Geometry check sheet. Reference: the model listing, model coordinates, mm. A direction names the side the tool comes from. Coordinates: 2 decimals unless noted, no trailing zeros. Write each loop counter-clockwise with the first axis right and the second up, starting at its lowest first coordinate (ties: lowest second). Pieces come first, ordered by that corner, then holes. Notation, with made-up numbers: M 30.25,76 L 40.25,76 A17 cw 40.25,100 Z; hole C 20,25 d7. An arc over 180 degrees is marked long. Write each question's results on one line, items separated by ' | '.
```python
from build123d import *

# Parameters (mm, degrees)
SKETCH_1_W                       = 400
SKETCH_1_H                       = 135
SKETCH_1_R                       = 3
SM_BASE_FLANGE_1_DEPTH           = 0.7
SM_EDGE_FLANGE_1_STRIP_W         = 3.2
SM_EDGE_FLANGE_1_STRIP_H         = 0.7
SM_EDGE_FLANGE_1_STRIP_CUT_DEPTH = 400
SM_EDGE_FLANGE_1_DEPTH           = 400
SM_EDGE_FLANGE_2_STRIP_W         = 3.2
SM_EDGE_FLANGE_2_STRIP_H         = 0.7
SM_EDGE_FLANGE_2_STRIP_CUT_DEPTH = 400
SM_EDGE_FLANGE_2_DEPTH           = 400


# Sheet-metal steps are written as plain solids
with BuildPart() as part:
    # Sketch 1 → 基体-法兰1 (new body)
    with BuildSketch(Plane(origin=(0, 0, 0), x_dir=(1, 0, 0), z_dir=(0, 1, 0))):
        Rectangle(SKETCH_1_W, SKETCH_1_H)
        with Locations(Location((-194.5, -60.5, 0), (0, 0, 270))):
            Circle(SKETCH_1_R, mode=Mode.SUBTRACT)
        with Locations(Location((-194.5, -10.5, 0), (0, 0, 270))):
            Circle(SKETCH_1_R, mode=Mode.SUBTRACT)
        with Locations(Location((-194.5, -0.5, 0), (0, 0, 270))):
            Circle(SKETCH_1_R, mode=Mode.SUBTRACT)
        with Locations(Location((-194.5, 49.5, 0), (0, 0, 270))):
            Circle(SKETCH_1_R, mode=Mode.SUBTRACT)
        with Locations(Location((0, -10.5, 0), (0, 0, 270))):
            Circle(SKETCH_1_R, mode=Mode.SUBTRACT)
        with Locations(Location((0, -0.5, 0), (0, 0, 270))):
            Circle(SKETCH_1_R, mode=Mode.SUBTRACT)
        with Locations(Location((194.5, -60.5, 0), (0, 0, 90))):
            Circle(SKETCH_1_R, mode=Mode.SUBTRACT)
        with Locations(Location((194.5, -10.5, 0), (0, 0, 90))):
            Circle(SKETCH_1_R, mode=Mode.SUBTRACT)
        with Locations(Location((194.5, -0.5, 0), (0, 0, 90))):
            Circle(SKETCH_1_R, mode=Mode.SUBTRACT)
        with Locations(Location((194.5, 49.5, 0), (0, 0, 90))):
            Circle(SKETCH_1_R, mode=Mode.SUBTRACT)
    extrude(amount=-SM_BASE_FLANGE_1_DEPTH)

    # 边线-法兰1 strip (across the edge) → 边线-法兰1 strip cut (cut)
    with BuildSketch(Plane(origin=(-200, -0.7, -67.5), x_dir=(0, 0, 1), z_dir=(1, 0, 0))):
        with Locations((-0.7, -0.35)):
            Rectangle(SM_EDGE_FLANGE_1_STRIP_W, SM_EDGE_FLANGE_1_STRIP_H)
    extrude(amount=SM_EDGE_FLANGE_1_STRIP_CUT_DEPTH, mode=Mode.SUBTRACT)

    # 边线-法兰1 section (across the edge) → 边线-法兰1 (add)
    with BuildSketch(Plane(origin=(-200, -0.7, -67.5), x_dir=(0, 0, 1), z_dir=(1, 0, 0))):
        with BuildLine():
            Line((0, 0.2), (0, 5.3))
            Line((0, 5.3), (0.7, 5.3))
            Line((0.7, 5.3), (0.7, 0.2))
            ThreePointArc((0.7, 0.2), (0.758578644, 0.058578644), (0.9, 0))
            Line((0.9, 0), (0.9, -0.7))
            ThreePointArc((0.9, -0.7), (0.263603897, -0.436396103), (0, 0.2))
        make_face()
    extrude(amount=SM_EDGE_FLANGE_1_DEPTH)

    # 边线-法兰2 strip (across the edge) → 边线-法兰2 strip cut (cut)
    with BuildSketch(Plane(origin=(200, -6, -67.5), x_dir=(0, 1, 0), z_dir=(-1, 0, 0))):
        with Locations((-0.7, -0.35)):
            Rectangle(SM_EDGE_FLANGE_2_STRIP_W, SM_EDGE_FLANGE_2_STRIP_H)
    extrude(amount=SM_EDGE_FLANGE_2_STRIP_CUT_DEPTH, mode=Mode.SUBTRACT)

    # 边线-法兰2 section (across the edge) → 边线-法兰2 (add)
    with BuildSketch(Plane(origin=(200, -6, -67.5), x_dir=(0, 1, 0), z_dir=(-1, 0, 0))):
        with BuildLine():
            Line((0, 0.2), (0, 5.3))
            Line((0, 5.3), (0.7, 5.3))
            Line((0.7, 5.3), (0.7, 0.2))
            ThreePointArc((0.7, 0.2), (0.758578644, 0.058578644), (0.9, 0))
            Line((0.9, 0), (0.9, -0.7))
            ThreePointArc((0.9, -0.7), (0.263603897, -0.436396103), (0, 0.2))
        make_face()
    extrude(amount=SM_EDGE_FLANGE_2_DEPTH)


solid = part.part
```
Q1. Depth check by flat-ended pin: P1, Ø3.5, axis at x = -194.5, z = -49.5, coming from the -Y side; P2, Ø4, axis at x = -44, z = -69, coming from the +Y side; P3, Ø9.5, axis at x = -194.5, z = 10.5, coming from the -Y side; P4, Ø3, axis at x = 47, y = -5, coming from the +Z side. Enter the tip coordinate at first touch or a pass-through.
Geometry check:
P1: passes through | P2: stops at y = -0.09 | P3: stops at y = -0.7 | P4: stops at z = -66.8
Q2. Sectioned sample at B-B on z = 39.5. Record the cut outline in (x, y).
Geometry check:
outline: M -200,-0.7 L 200,-0.7 L 200,0 L -200,0 Z
Q3. Scan lines: probe 1 along X at (y, z) = (-0.4, 10.5); probe 2 along X at (y, z) = (-0.5, 60.5); probe 3 along Z at (x, y) = (194.5, -0.25). Record each from-to range of solid material in increasing order.
Geometry check:
probe 1: x = -200 to -197.5, -191.5 to -3, 3 to 191.5, 197.5 to 200 | probe 2: x = -200 to -197.5, -191.5 to 191.5, 197.5 to 200 | probe 3: z = -67.22 to -52.5, -46.5 to -2.5, 3.5 to 7.5, 13.5 to 57.5, 63.5 to 67.5
Q4. Sectioned sample at C-C on y = -3.9. Record the cut outline in (x, z), and give its area (3 significant figures).
Geometry check:
outline: M -200,-67.5 L 200,-67.5 L 200,-66.8 L -200,-66.8 Z | area: 280 mm2
Q5. Access from +Z, -Z, +X, -X, +Y, -Y to the whole of each face (thin tool, end or side, straight path). Record for faces 1 (the flat face through (-3, -0.7, -15)), 2 (the flat face through (-3, 0, -15)).
Geometry check:
face 1: +Z, +X, -X, -Y | face 2: +Z, -Z, +X, -X, +Y
Q6. Sectioned sample at A-A on x = -9.5. Record the cut outline in (y, z).
Geometry check:
outline: M -6,-72.8 L -5.3,-72.8 L -5.3,-67.7 A0.2 cw -5.1,-67.5 L -0.9,-67.5 A0.9 ccw 0,-66.6 L 0,67.5 L -0.7,67.5 L -0.7,-66.6 A0.2 cw -0.9,-66.8 L -5.1,-66.8 A0.9 ccw -6,-67.7 Z
